```python
from build123d import *


with BuildPart() as f1:
    # F0 (on Front) → F1 (revolve)
    with BuildSketch(Plane.XZ):
        with BuildLine():
            Line((-32.440171, 9.240504), (-32.521368, 10.240504))
            Line((-32.521368, 10.240504), (-36.5, 10.240504))
            Line((-36.5, 10.240504), (-36.5, 59.240504))
            Line((-36.5, 59.240504), (-33.220742, 35.719246))
            Line((-33.220742, 35.719246), (-32.230321, 35.857327))
            Line((-32.230321, 35.857327), (-35.509579, 59.378585))
            Line((-35.509579, 59.378585), (-35.588887, 59.947439))
            ThreePointArc((-35.588887, 59.947439), (-35.762638, 60.261366), (-36.101928, 60.378081))
            Line((-36.101928, 60.378081), (-37.01783, 60.345398))
            ThreePointArc((-37.01783, 60.345398), (-37.359802, 60.192909), (-37.5, 59.845716))
            Line((-37.5, 59.845716), (-37.5, 59.240504))
            Line((-37.5, 59.240504), (-37.5, 10.240504))
            Line((-37.5, 10.240504), (-72.440171, 10.240504))
            ThreePointArc((-72.440171, 10.240504), (-78.804132, 12.876543), (-81.440171, 19.240504))
            Line((-81.440171, 19.240504), (-81.440171, 64.240504))
            Line((-81.440171, 64.240504), (-82.440171, 64.240504))
            Line((-82.440171, 64.240504), (-82.440171, 19.240504))
            ThreePointArc((-82.440171, 19.240504), (-79.511239, 12.169436), (-72.440171, 9.240504))
            Line((-72.440171, 9.240504), (-32.440171, 9.240504))
        make_face()
    revolve(axis=Axis((0, 0, 34.240504), (0, 0, 1)))


solid = f1.part
```
For this review, take the finished solid that the model builds, in its own axes (mm). A direction names the side the tool comes from. Give positions to 0.01 mm unless a question says otherwise; leave off trailing zeros. Write each loop counter-clockwise with the first axis right and the second up, starting at its lowest first coordinate (ties: lowest second). Pieces come first, ordered by that corner, then holes. Notation, with made-up numbers: M -14.5,-31.5 L 9.5,-31.5 A27 cw 9.5,-10.5 Z; hole C -27,53 d4. An arc over 180 degrees is marked long. Answer as a JSON object with one key per item and string values. Group by question number.
Item 1: Consider section B-B on z = 23. Write out the cut boundary in (x, y), plus the area to 3 significant figures.
Item 2: For probe 1 along X at (y, z) = (-1, 26); probe 2 along Y at (x, z) = (0, 34.5); probe 3 along Y at (x, z) = (0, 45), list the stretches that pass through material, from the lowest coordinate up. Write a range as [from, to].
Item 3: Tool access review of faces 1 (the cylindrical face through (-77.68, -24.46, 42.06)), 2 (the flat face through (-80, -19, 64.241)), 3 (the cylindrical face through (7.912, 35.632, 35.084)): name each direction out of +Z, -Z, +X, -X, +Y, -Y from which nothing blocks a thin tool from reaching the whole face with its end or side.
Item 4: Draft analysis for pull direction Y (two halves, no side actions). For faces 4 (the flat face through (-31, 15, 9.241)), 5 (the cylindrical face through (17.87, 80.48, 41.43)), 6 (the conical face through (-32.534, -10.245, 42.088)), 7 (the cylindrical face through (4.88, -37.18, 34.7)), state which applies: +Y half, -Y half, draft (parallel to the pull), parting line (faces both ways), or undercut.
Item 5: For pin 1 Ø12 at (y, z) = (-51, 33) entering from +X; pin 2 Ø3 at (x, z) = (15, 33.5) entering from +Y; pin 3 Ø8 at (x, z) = (-10, 52.5) entering from -Y, all flat-tipped, find the tip position at first contact; note any pin that passes through.
Item 6: Consider section A-A on z = 50.5. Write out the cut boundary in (x, y), plus the area to 3 significant figures.
Check result:
{
 "1": {"outline": "C 0,0 d164.88; C 0,0 d75; hole C 0,0 d162.88; hole C 0,0 d73", "area": "747 mm^2"},
 "2": {"probe 1": "x = [-82.43, -81.43], [-37.49, -36.49], [36.49, 37.49], [81.43, 82.43]", "probe 2": "y = [-82.44, -81.44], [-37.5, -36.5], [36.5, 37.5], [81.44, 82.44]", "probe 3": "y = [-82.44, -81.44], [-37.5, -36.5], [-34.51, -33.5], [33.5, 34.51], [36.5, 37.5], [81.44, 82.44]"},
 "3": {"face 1": "+Z", "face 2": "+Z, +X, -X, +Y, -Y", "face 3": "none"},
 "4": {"face 4": "draft", "face 5": "parting line", "face 6": "undercut", "face 7": "undercut"},
 "5": {"pin 1": "stops at x = 69.08", "pin 2": "stops at y = 81.33", "pin 3": "stops at y = -82.22"},
 "6": {"outline": "C 0,0 d164.88; C 0,0 d75; C 0,0 d70.56; hole C 0,0 d162.88; hole C 0,0 d73; hole C 0,0 d68.54", "area": "968 mm^2"}
}
